Read the model definition and answer for the solid it produces. Units are mm, in the model's axes. A direction names the side the tool comes from. Round coordinates to 2 decimals unless told otherwise and drop trailing zeros. Order: outer loops, then holes, each group sorted by start corner. A loop starts at its lowest first (then second) coordinate and runs counter-clockwise, first axis right, second up. Notation, with made-up numbers: (-37.75, 54) -> (8.25, 54) arc R22 cw to (8.25, 66) -> close; hole circle Ø1 at (22.25, 56.25). An arc over 180 degrees is marked (long way). Answer as a JSON object with one key per item and string values. Group by question number.
Item 1: Section D-D, the plane x = -19.5 is taken. Write down the section's boundary in (y, z), plus the area to 3 significant figures.
Item 2: Section B-B, the plane x = 0 is taken. Write down the section's boundary in (y, z), plus the area to 3 significant figures.
Item 3: Section C-C, the plane z = 5.25 is taken. Write down the section's boundary in (x, y).
Item 4: Consider probe 1 along Y at (x, z) = (0, 3.15); probe 2 along Y at (x, z) = (5, 6.5); probe 3 along Z at (x, y) = (-17, 8). Determine where each line is inside the solid, lowest interval first. Write a range as from..to.
Item 5: Given P1, Ø5, axis at x = -15, y = 2, coming from the +Z side; P2, Ø0.9, axis at y = 10.5, z = 5, coming from the -X side; P3, Ø3.5, axis at x = -1, z = 3, coming from the -Y side; P4, Ø7.5, axis at x = 0, y = 8.5, coming from the +Z side, each flat-ended and moving along its own axis, determine where each tip first touches the part or whether it passes through.
Item 6: For faces 1 (the flat face through (3.5, 9, 5)), 2 (the flat face through (-20, -41.5, 3.5)), 3 (the flat face through (-6.5, 9, 5)), 4 (the flat face through (-3, 5.5, 3)), determine the directions among +Z, -Z, +X, -X, +Y, -Y from which every point of the face is accessible in a straight line to the end or side of a thin tool.
Item 7: Section A-A, the plane y = 9 is taken. Write down the section's boundary in (x, z).
Item 8: The mould has two halves that part along X. Classify faces 5 (the flat face through (-17.4, -41.4, 2)), 6 (the flat face through (-20, -41.5, 0.5)), 7 (the flat face through (0, 7, 4)): pulls with the +X half, pulls with the -X half, needs draft (parallel to the pull), parting line crosses it, or undercut.
from build123d import *

# Parameters (mm, degrees)
SKETCH2_W           = 18.5
SKETCH2_H           = 7
SKETCH2_R           = 1.45
BOSS_EXTRUDE2_DEPTH = 4
SKETCH4_W           = 3
SKETCH4_H           = 7
BOSS_EXTRUDE3_DEPTH = 7
SKETCH5_W           = 2
SKETCH5_H           = 7
SKETCH5_W_2         = 6
SKETCH5_H_2         = 54.5
BOSS_EXTRUDE4_DEPTH = 4
FILLET1_DEPTH       = 4
CHAMFER1_SIZE       = 9
CHAMFER6_SIZE       = 1


with BuildPart() as part:
    # Sketch2 → Boss-Extrude2 (new body)
    with BuildSketch(Plane.XY):
        with Locations((-5.75, 9)):
            Rectangle(SKETCH2_W, SKETCH2_H)
        with Locations((0, 9)):
            Circle(SKETCH2_R, mode=Mode.SUBTRACT)
    extrude(amount=BOSS_EXTRUDE2_DEPTH)

    # Sketch4 → Boss-Extrude3 (add)
    with BuildSketch(Plane.XY):
        with Locations((5, 9)):
            Rectangle(SKETCH4_W, SKETCH4_H)
        with Locations((-5, 9)):
            Rectangle(SKETCH4_W, SKETCH4_H)
    extrude(amount=BOSS_EXTRUDE3_DEPTH)

    # Sketch5 → Boss-Extrude4 (add)
    with BuildSketch(Plane.XY):
        with Locations((-16, 9)):
            Rectangle(SKETCH5_W, SKETCH5_H)
        with Locations((-20, -14.75)):
            Rectangle(SKETCH5_W_2, SKETCH5_H_2)
    extrude(amount=BOSS_EXTRUDE4_DEPTH)

    # Fillet1: read off the stored shape, not the designer's step
    # Fillet1 outline → Fillet1 (add)
    with BuildSketch(Plane.XY):
        with BuildLine():
            add(Edge.make_bspline(
                [(-12, 5.5), (-17, 5.5), (-17, 0.5)],
                knots=[0, 0, 0, 1, 1, 1], degree=2, weights=[1, 0.000353553, 1]))
            Line((-12, 5.5), (-17, 5.5))
            Line((-17, 5.5), (-17, 0.5))
        make_face()
    extrude(amount=FILLET1_DEPTH)

    # Chamfer1
    chamfer1_edges = [part.edges().sort_by_distance(p)[0] for p in [
        (-23, 12.5, 2),
    ]]
    chamfer(chamfer1_edges, length=CHAMFER1_SIZE)

    # Chamfer6
    chamfer6_edges = [part.edges().sort_by_distance(p)[0] for p in [
        (-20, -42, 4),
        (-23, -42, 2),
        (-17, -42, 2),
        (-20, -42, 0),
    ]]
    chamfer(chamfer6_edges, length=CHAMFER6_SIZE)


solid = part.part
Values found:
{
 "1": {"outline": "(-42, 1) -> (-41, 0) -> (7, 0) -> (7, 4) -> (-41, 4) -> (-42, 3) -> close", "area": "195 mm2"},
 "2": {"outline": "(5.5, 0) -> (7.55, 0) -> (7.55, 4) -> (5.5, 4) -> close; (10.45, 0) -> (12.5, 0) -> (12.5, 4) -> (10.45, 4) -> close", "area": "16.4 mm2"},
 "3": {"outline": "(-6.5, 5.5) -> (-3.5, 5.5) -> (-3.5, 12.5) -> (-6.5, 12.5) -> close; (3.5, 5.5) -> (6.5, 5.5) -> (6.5, 12.5) -> (3.5, 12.5) -> close"},
 "4": {"probe 1": "5.5..7.55, 10.45..12.5", "probe 2": "5.5..12.5", "probe 3": "0..4"},
 "5": {"P1": "z = 4", "P2": "x = -6.5", "P3": "y = 5.5", "P4": "z = 7"},
 "6": {"face 1": "+Z, +Y, -Y", "face 2": "+Z, +X, -X, -Y", "face 3": "+Z, -X, +Y, -Y", "face 4": "+Z, -Z, +X, -Y"},
 "7": {"outline": "(-17.5, 0) -> (-1.45, 0) -> (-1.45, 4) -> (-3.5, 4) -> (-3.5, 7) -> (-6.5, 7) -> (-6.5, 4) -> (-17.5, 4) -> close; (1.45, 0) -> (6.5, 0) -> (6.5, 7) -> (3.5, 7) -> (3.5, 4) -> (1.45, 4) -> close"},
 "8": {"face 5": "pulls with the +X half", "face 6": "needs draft", "face 7": "undercut"}
}
